from build123d import *

# Parameters (mm, degrees)
F0_W     = 63.5
F0_H     = 25.4
F0_W_2   = 54.6053671278
F0_H_2   = 16.0604021512
F1_DEPTH = 5.08
F0_W_3   = 1.2807164436
F0_H_3   = 8.4517414633
F2_DEPTH = 3.175
F3_R     = 2.54
F4_DEPTH = 25.4
F5_DEPTH = 3.175


with BuildPart() as f1:
    # F0 (on Front) → F1 (new body)
    with BuildSketch(Plane.XZ):
        with Locations((31.75, 12.7)):
            Rectangle(F0_W, F0_H)
        with Locations((31.5367903095, 11.9723000098)):
            Rectangle(F0_W_2, F0_H_2, mode=Mode.SUBTRACT)
    extrude(amount=F1_DEPTH)

    # F0 (on Front) → F2 (join)
    with BuildSketch(Plane.XZ):
        with Locations((31.5367903095, 11.9723000098)):
            Rectangle(F0_W_2, F0_H_2)
        with Locations((22.7084914528, 10.7061468506)):
            Rectangle(F0_W_3, F0_H_3, mode=Mode.SUBTRACT)
        Polygon((15.4202525004, 11.2996194994), (15.4202525004, 6.480276119), (14.1099241159, 6.480276119), (14.1099241159, 17.7550226141), (20.3950585705, 17.7550226141), (20.3950585705, 16.5902862723), (15.4202525004, 16.5902862723), (15.4202525004, 12.4643558412), (20.0940038381, 12.4643558412), (20.0940038381, 11.2996194994), align=None, mode=Mode.SUBTRACT)
        with BuildLine():
            Line((29.4094269108, 6.480276119), (27.9140238957, 6.480276119))
            Line((27.9140238957, 6.480276119), (24.7060636322, 14.9320175823))
            Line((24.7060636322, 14.9320175823), (26.0780835603, 14.9320175823))
            Line((26.0780835603, 14.9320175823), (27.8992179252, 9.9201965861))
            add(Edge.make_bspline(
                [(27.8992179252, 9.9201965861), (28.5161333605, 8.1607537647), (28.6247104771, 7.6376094755)],
                knots=[0, 0, 0, 1, 1, 1], degree=2))
            Line((28.6247104771, 7.6376094755), (28.6864020207, 7.6376094755))
            add(Edge.make_bspline(
                [(28.6864020207, 7.6376094755), (28.7703025199, 8.0447736628), (29.2218846185, 9.3291915991)],
                knots=[0, 0, 0, 1, 1, 1], degree=2))
            add(Edge.make_bspline(
                [(29.2218846185, 9.3291915991), (29.6734667171, 10.6136095353), (31.2453672462, 14.9320175823)],
                knots=[0, 0, 0, 1, 1, 1], degree=2))
            Line((31.2453672462, 14.9320175823), (32.6173871743, 14.9320175823))
            Line((32.6173871743, 14.9320175823), (29.4094269108, 6.480276119))
        make_face(mode=Mode.SUBTRACT)
        with BuildLine():
            add(Edge.make_bspline(
                [(39.006163422, 6.4531318398), (38.4015862954, 6.3248134293), (37.5453076713, 6.3248134293)],
                knots=[0, 0, 0, 1, 1, 1], degree=2))
            add(Edge.make_bspline(
                [(37.5453076713, 6.3248134293), (35.6723524098, 6.3248134293), (34.5878150745, 7.4673408154)],
                knots=[0, 0, 0, 1, 1, 1], degree=2))
            add(Edge.make_bspline(
                [(34.5878150745, 7.4673408154), (33.5032777393, 8.6098682015), (33.5032777393, 10.635818491)],
                knots=[0, 0, 0, 1, 1, 1], degree=2))
            add(Edge.make_bspline(
                [(33.5032777393, 10.635818491), (33.5032777393, 12.6815100744), (34.5100837297, 13.8844951732)],
                knots=[0, 0, 0, 1, 1, 1], degree=2))
            add(Edge.make_bspline(
                [(34.5100837297, 13.8844951732), (35.5168897201, 15.087480272), (37.214640998, 15.087480272)],
                knots=[0, 0, 0, 1, 1, 1], degree=2))
            add(Edge.make_bspline(
                [(37.214640998, 15.087480272), (38.8013474975, 15.087480272), (39.7267206504, 14.0424255246)],
                knots=[0, 0, 0, 1, 1, 1], degree=2))
            add(Edge.make_bspline(
                [(39.7267206504, 14.0424255246), (40.6520938033, 12.9973707773), (40.6520938033, 11.2848135289)],
                knots=[0, 0, 0, 1, 1, 1], degree=2))
            Line((40.6520938033, 11.2848135289), (40.6520938033, 10.4754204778))
            Line((40.6520938033, 10.4754204778), (34.830879756, 10.4754204778))
            add(Edge.make_bspline(
                [(34.830879756, 10.4754204778), (34.8703623439, 8.9874204479), (35.5835165871, 8.2162761538)],
                knots=[0, 0, 0, 1, 1, 1], degree=2))
            add(Edge.make_bspline(
                [(35.5835165871, 8.2162761538), (36.2966708303, 7.4451318597), (37.5921932444, 7.4451318597)],
                knots=[0, 0, 0, 1, 1, 1], degree=2))
            add(Edge.make_bspline(
                [(37.5921932444, 7.4451318597), (38.9568101872, 7.4451318597), (40.2893475274, 8.0151617219)],
                knots=[0, 0, 0, 1, 1, 1], degree=2))
            Line((40.2893475274, 8.0151617219), (40.2893475274, 6.8726343358))
            add(Edge.make_bspline(
                [(40.2893475274, 6.8726343358), (39.6107405486, 6.5814502503), (39.006163422, 6.4531318398)],
                knots=[0, 0, 0, 1, 1, 1], degree=2))
        make_face(mode=Mode.SUBTRACT)
        with BuildLine():
            add(Edge.make_bspline(
                [(51.2531686432, 10.1817687306), (51.7812482558, 9.6265448389), (51.7812482558, 8.7850721852)],
                knots=[0, 0, 0, 1, 1, 1], degree=2))
            add(Edge.make_bspline(
                [(51.7812482558, 8.7850721852), (51.7812482558, 7.6055298729), (50.902760676, 6.9651716511)],
                knots=[0, 0, 0, 1, 1, 1], degree=2))
            add(Edge.make_bspline(
                [(50.902760676, 6.9651716511), (50.0242730961, 6.3248134293), (48.4350989348, 6.3248134293)],
                knots=[0, 0, 0, 1, 1, 1], degree=2))
            add(Edge.make_bspline(
                [(48.4350989348, 6.3248134293), (46.7546212891, 6.3248134293), (45.8144421658, 6.8578283654)],
                knots=[0, 0, 0, 1, 1, 1], degree=2))
            Line((45.8144421658, 6.8578283654), (45.8144421658, 8.0447736628))
            add(Edge.make_bspline(
                [(45.8144421658, 8.0447736628), (46.4239546158, 7.7363159452), (47.1210690577, 7.5598781307)],
                knots=[0, 0, 0, 1, 1, 1], degree=2))
            add(Edge.make_bspline(
                [(47.1210690577, 7.5598781307), (47.8181834996, 7.3834403162), (48.4671785375, 7.3834403162)],
                knots=[0, 0, 0, 1, 1, 1], degree=2))
            add(Edge.make_bspline(
                [(48.4671785375, 7.3834403162), (49.4690492044, 7.3834403162), (50.0082332948, 7.7030025117)],
                knots=[0, 0, 0, 1, 1, 1], degree=2))
            add(Edge.make_bspline(
                [(50.0082332948, 7.7030025117), (50.5474173852, 8.0225647072), (50.5474173852, 8.6789627303)],
                knots=[0, 0, 0, 1, 1, 1], degree=2))
            add(Edge.make_bspline(
                [(50.5474173852, 8.6789627303), (50.5474173852, 9.1724950785), (50.120511904, 9.5229030458)],
                knots=[0, 0, 0, 1, 1, 1], degree=2))
            add(Edge.make_bspline(
                [(50.120511904, 9.5229030458), (49.6936064228, 9.873311013), (48.4499049053, 10.3520373908)],
                knots=[0, 0, 0, 1, 1, 1], degree=2))
            add(Edge.make_bspline(
                [(48.4499049053, 10.3520373908), (47.270362593, 10.7912811807), (46.7731287522, 11.1194801923)],
                knots=[0, 0, 0, 1, 1, 1], degree=2))
            add(Edge.make_bspline(
                [(46.7731287522, 11.1194801923), (46.2758949114, 11.4476792038), (46.0328302299, 11.8634802072)],
                knots=[0, 0, 0, 1, 1, 1], degree=2))
            add(Edge.make_bspline(
                [(46.0328302299, 11.8634802072), (45.7897655484, 12.2792812106), (45.7897655484, 12.856714058)],
                knots=[0, 0, 0, 1, 1, 1], degree=2))
            add(Edge.make_bspline(
                [(45.7897655484, 12.856714058), (45.7897655484, 13.8906643275), (46.6312382021, 14.4890722998)],
                knots=[0, 0, 0, 1, 1, 1], degree=2))
            add(Edge.make_bspline(
                [(46.6312382021, 14.4890722998), (47.4727108558, 15.087480272), (48.9360342683, 15.087480272)],
                knots=[0, 0, 0, 1, 1, 1], degree=2))
            add(Edge.make_bspline(
                [(48.9360342683, 15.087480272), (50.3006512111, 15.087480272), (51.6060442722, 14.5322563802)],
                knots=[0, 0, 0, 1, 1, 1], degree=2))
            Line((51.6060442722, 14.5322563802), (51.1495268501, 13.4909031255))
            add(Edge.make_bspline(
                [(51.1495268501, 13.4909031255), (49.8786810534, 14.0140474146), (48.8447307839, 14.0140474146)],
                knots=[0, 0, 0, 1, 1, 1], degree=2))
            add(Edge.make_bspline(
                [(48.8447307839, 14.0140474146), (47.9341636014, 14.0140474146), (47.4714770249, 13.7290324835)],
                knots=[0, 0, 0, 1, 1, 1], degree=2))
            add(Edge.make_bspline(
                [(47.4714770249, 13.7290324835), (47.0087904485, 13.4440175524), (47.0087904485, 12.943082219)],
                knots=[0, 0, 0, 1, 1, 1], degree=2))
            add(Edge.make_bspline(
                [(47.0087904485, 12.943082219), (47.0087904485, 12.6025448987), (47.1827606012, 12.3644155407)],
                knots=[0, 0, 0, 1, 1, 1], degree=2))
            add(Edge.make_bspline(
                [(47.1827606012, 12.3644155407), (47.356730754, 12.1262861826), (47.7416859856, 11.9103657803)],
                knots=[0, 0, 0, 1, 1, 1], degree=2))
            add(Edge.make_bspline(
                [(47.7416859856, 11.9103657803), (48.1266412172, 11.6944453779), (49.2222830303, 11.2848135289)],
                knots=[0, 0, 0, 1, 1, 1], degree=2))
            add(Edge.make_bspline(
                [(49.2222830303, 11.2848135289), (50.7250890306, 10.7369926224), (51.2531686432, 10.1817687306)],
                knots=[0, 0, 0, 1, 1, 1], degree=2))
        make_face(mode=Mode.SUBTRACT)
        with BuildLine():
            add(Edge.make_bspline(
                [(22.1754765167, 16.5779479636), (21.9595561144, 16.7901668734), (21.9595561144, 17.2220076781)],
                knots=[0, 0, 0, 1, 1, 1], degree=2))
            add(Edge.make_bspline(
                [(21.9595561144, 17.2220076781), (21.9595561144, 17.661251468), (22.1754765167, 17.8660673925)],
                knots=[0, 0, 0, 1, 1, 1], degree=2))
            add(Edge.make_bspline(
                [(22.1754765167, 17.8660673925), (22.3913969191, 18.070883317), (22.7171282689, 18.070883317)],
                knots=[0, 0, 0, 1, 1, 1], degree=2))
            add(Edge.make_bspline(
                [(22.7171282689, 18.070883317), (23.0255859865, 18.070883317), (23.2489093741, 17.8623658999)],
                knots=[0, 0, 0, 1, 1, 1], degree=2))
            add(Edge.make_bspline(
                [(23.2489093741, 17.8623658999), (23.4722327617, 17.6538484827), (23.4722327617, 17.2220076781)],
                knots=[0, 0, 0, 1, 1, 1], degree=2))
            add(Edge.make_bspline(
                [(23.4722327617, 17.2220076781), (23.4722327617, 16.7901668734), (23.2489093741, 16.5779479636)],
                knots=[0, 0, 0, 1, 1, 1], degree=2))
            add(Edge.make_bspline(
                [(23.2489093741, 16.5779479636), (23.0255859865, 16.3657290539), (22.7171282689, 16.3657290539)],
                knots=[0, 0, 0, 1, 1, 1], degree=2))
            add(Edge.make_bspline(
                [(22.7171282689, 16.3657290539), (22.3913969191, 16.3657290539), (22.1754765167, 16.5779479636)],
                knots=[0, 0, 0, 1, 1, 1], degree=2))
        make_face(mode=Mode.SUBTRACT)
        Polygon((42.5053077709, 17.7550226141), (43.9390192425, 17.7550226141), (43.6305615249, 13.6833807413), (42.8211684738, 13.6833807413), align=None, mode=Mode.SUBTRACT)
    extrude(amount=F2_DEPTH)

    # F3 (on Front) → F4 (cut)
    with BuildSketch(Plane.XZ):
        with Locations((4.3997538427, 11.8095606944)):
            Circle(F3_R)
    extrude(amount=F4_DEPTH, mode=Mode.SUBTRACT)

    # F5 (add): a face of the model
    f5_faces = [f1.faces().sort_by_distance(p)[0] for p in [
        (31.8480546153, -3.175, 12.0163754406),
    ]]
    extrude(f5_faces, amount=-F5_DEPTH)


solid = f1.part
Can you work these out from the model? Positions are in its coordinate system, mm. A direction names the side the tool comes from. Coordinates: 2 decimals unless noted, no trailing zeros. Write each loop counter-clockwise with the first axis right and the second up, starting at its lowest first coordinate (ties: lowest second). Pieces come first, ordered by that corner, then holes. Notation, with made-up numbers: (-14.75, -27) -> (-0.75, -27) arc R21 cw to (-0.75, 11) -> close; hole circle Ø10 at (-3.75, -5.5). An arc over 180 degrees is marked (long way). Write each question's results on one line, items separated by ' | '. Start each with the question number.
Q1. Imagine slicing it at D-D (x = 8). Write out the boundary of the cut face in (y, z) (1 decimal).
Q2. If I drill on probe 1 along X at (y, z) = (-4.7, 19.75); probe 2 along Z at (x, y) = (43, -2.1); probe 3 along Z at (x, y) = (29.5, -4.75), over which ranges is the centre line in solid material (lowest first)?
Q3. Imagine slicing it at C-C (z = 4.5). Write out the boundary of the cut face in (x, y) (3 decimals), then the cut area to 3 significant figures.
Q4. Imagine slicing it at B-B (x = 18). Write out the boundary of the cut face in (y, z) (1 decimal).
Q5. Imagine slicing it at A-A (y = -4.4). Write out the boundary of the cut face in (x, z).
Q6. On a 3-axis mill with a long thin cutter (end or side, diameter ignored), from which of +Z, -Z, +X, -X, +Y, -Y can I reach the whole of each face in a straight line? I mean faces 1 (the face through (15.42, -2, 9)), 2 (the face through (31, -4, 20.003)), 3 (the face through (31, -5.08, 21)). Say none if no direction works.
Q7. We'd pull the mould along X, two halves only. Please class faces 4 (the face through (63.5, -3, 13)), 5 (the face through (31, -3, 25.4)), 6 (the face through (23.349, -2, 11)): +X half, -X half, draft (parallel to the pull), parting line (faces both ways), or undercut.
Taken from the geometry:
1) outline: (-5.1, 0) -> (0, 0) -> (0, 25.4) -> (-5.1, 25.4) -> (-5.1, 20) -> (-3.2, 20) -> (-3.2, 3.9) -> (-5.1, 3.9) -> close
2) probe 1: x = 0 to 4.23, 58.84 to 63.5 | probe 2: z = 0 to 13.68, 17.76 to 25.4 | probe 3: z = 0 to 3.94, 20 to 25.4
3) outline: (0, -5.08) -> (4.234, -5.08) -> (4.234, -3.175) -> (58.839, -3.175) -> (58.839, -5.08) -> (63.5, -5.08) -> (63.5, 0) -> (0, 0) -> close | area: 219 mm^2
4) outline: (-5.1, 0) -> (0, 0) -> (0, 11.3) -> (-3.2, 11.3) -> (-3.2, 3.9) -> (-5.1, 3.9) -> close; (-5.1, 20) -> (-3.2, 20) -> (-3.2, 17.8) -> (0, 17.8) -> (0, 25.4) -> (-5.1, 25.4) -> close; (-3.2, 12.5) -> (0, 12.5) -> (0, 16.6) -> (-3.2, 16.6) -> close
5) outline: (0, 0) -> (63.5, 0) -> (63.5, 25.4) -> (0, 25.4) -> close; hole (4.23, 3.94) -> (58.84, 3.94) -> (58.84, 20) -> (4.23, 20) -> (4.23, 14.34) arc R2.54 ccw to (4.23, 9.27) -> close
6) face 1: +Y, -Y | face 2: -Y | face 3: +Z, -Z, +X, -X, -Y
7) face 4: +X half | face 5: draft | face 6: undercut
